Work out the finished part from the listing and answer in its coordinate system (mm). A direction names the side the tool comes from. Coordinates: 2 decimals unless noted, no trailing zeros. Loops run counter-clockwise (first coordinate to the right, second up) from the corner with the lowest first, then second, coordinate; pieces in that order, holes last. Notation, with made-up numbers: (13.25, 26) -> (46.25, 26) arc R6 cw to (46.25, 33) -> close; hole circle Ø9 at (-36, 35.5). An arc over 180 degrees is marked (long way). Use a Markdown table: item, result.
from build123d import *

# Parameters (mm, degrees)
SKETCH_1_R                   = 8
EXTRUDE_1_DEPTH              = 32
SKETCH_2_W                   = 1
SKETCH_2_H                   = 10
CUT_EXTRUDE_2_DEPTH          = 9.25
HOLE_WIZARD_M8_1_D           = 6.8
HOLE_WIZARD_M8_1_DEPTH       = 19.75
HOLE_WIZARD_M8_1_CBORE_D     = 8
HOLE_WIZARD_M8_1_CBORE_DEPTH = 16
HOLE_WIZARD_M8_1_TIP         = 2.042926105
SKETCH_4_R                   = 5
EXTRUDE_3_DEPTH              = 12
CHAMFER_1_SIZE               = 0.5
SKETCH_5_W                   = 1.5
SKETCH_5_H                   = 0.069985642


with BuildPart() as part:
    # 草图1 → 拉伸1 (new body)
    with BuildSketch(Plane.XY):
        Circle(SKETCH_1_R)
    extrude(amount=EXTRUDE_1_DEPTH)

    # 草图2 → 拉伸2 (cut, symmetric)
    with BuildSketch(Plane(origin=(0, 0, 0), x_dir=(1, 0, 0), z_dir=(0, 1, 0))):
        with Locations((-7.5, -16)):
            Rectangle(SKETCH_2_W, SKETCH_2_H)
        with Locations((7.5, -16)):
            Rectangle(SKETCH_2_W, SKETCH_2_H)
    extrude(amount=CUT_EXTRUDE_2_DEPTH, both=True, mode=Mode.SUBTRACT)

    # M8 螺纹孔1
    with Locations(Plane(origin=(0, 0, 0), x_dir=(-1, 0, 0), z_dir=(0, 0, -1))):
        with Locations((0, 0)):
            CounterBoreHole(HOLE_WIZARD_M8_1_D / 2, HOLE_WIZARD_M8_1_CBORE_D / 2, HOLE_WIZARD_M8_1_CBORE_DEPTH, depth=HOLE_WIZARD_M8_1_DEPTH)
            with Locations((0, 0, -(HOLE_WIZARD_M8_1_DEPTH + HOLE_WIZARD_M8_1_TIP / 2))):  # 118° drill point
                Cone(0, HOLE_WIZARD_M8_1_D / 2, HOLE_WIZARD_M8_1_TIP, mode=Mode.SUBTRACT)

    # 草图4 → 拉伸3 (add)
    with BuildSketch(Plane.XY.offset(32)):
        Circle(SKETCH_4_R)
    extrude(amount=EXTRUDE_3_DEPTH)

    # 倒角1
    chamfer_1_edges = [part.edges().sort_by_distance(p)[0] for p in [
        (-5, 0, 44),
    ]]
    chamfer(chamfer_1_edges, length=CHAMFER_1_SIZE)

    # 草图5 → 切除-旋转1 (revolve, cut)
    with BuildSketch(Plane(origin=(0, 0, 0), x_dir=(0, 0, -1), z_dir=(1, 0, 0)), mode=Mode.PRIVATE) as cut_revolve_1_sk:
        with Locations((-32.75, 4.465007179)):
            Rectangle(SKETCH_5_W, SKETCH_5_H)
    revolve(cut_revolve_1_sk.sketch.rotate(Axis((0, 0, 32), (0, 0, -1)), 90), axis=Axis((0, 0, 32), (0, 0, -1)), mode=Mode.SUBTRACT)


solid = part.part
Q1. Section B-B on y = 1.5 is taken. State how many separate pieces and enclosed holes the cut face has, and give its area (3 significant figures).
Solved:
| item | result |
|---|---|
| separate pieces | 1 |
| enclosed holes | 2 |
| area | 454 mm² |
Q2. For faces 5 (the cylindrical face through (0.867, -3.905, 7.888)), 6 (the cylindrical face through (-1.08, -4.88, 37.67)), 7 (the flat face through (-4, -2, 0)), 8 (the flat face through (7.4, 0.1, 21)), 9 (the flat face through (-7.4, -0.1, 21)), determine the directions among +Z, -Z, +X, -X, +Y, -Y from which every point of the face is accessible in a straight line to the end or side of a thin tool.
Solved:
| item | result |
|---|---|
| face 5 | -Z |
| face 6 | +Z |
| face 7 | -Z, +X, -X, +Y, -Y |
| face 8 | +X, +Y, -Y |
| face 9 | -X, +Y, -Y |
Q3. Consider line 1 (Y direction, x = 0, z = 17.2); line 2 (Y direction, x = 0, z = 4); line 3 (Z direction, x = 6, y = 1.25). Determine where each line is inside the solid, lowest interval first. Write a range as [from, to].
Solved:
| item | result |
|---|---|
| line 1 | [-8, -3.4], [3.4, 8] |
| line 2 | [-8, -4], [4, 8] |
| line 3 | [0, 32] |
Q4. Section C-C on z = 38 is taken. Determine the outline of the cut face in (x, y).
Solved:
| item | result |
|---|---|
| outline | circle Ø10 at (0, 0) |
Q5. Determine the mould class of faces 1 (the flat face through (-7.4, -0.1, 11)), 2 (the cylindrical face through (-6.349, -4.868, 15.776)), 3 (the flat face through (7, 0, 16)), 4 (the cylindrical face through (-0.74, -3.32, 17.9)) for opening direction X: pulls with the +X half, pulls with the -X half, needs draft (parallel to the pull), parting line crosses it, or undercut.
Solved:
| item | result |
|---|---|
| face 1 | needs draft |
| face 2 | parting line crosses it |
| face 3 | pulls with the +X half |
| face 4 | undercut |
Q6. Section A-A on z = 12.5 is taken. Determine the outline of the cut face in (x, y).
Solved:
| item | result |
|---|---|
| outline | (-7, -3.87) arc R8 ccw to (7, -3.87) -> (7, 3.87) arc R8 ccw to (-7, 3.87) -> close; hole circle Ø8 at (0, 0) |
Q7. Given pin 1 Ø2 at (x, z) = (5.5, 9) entering from +Y; pin 2 Ø6.5 at (x, y) = (0, 0) entering from -Z; pin 3 Ø4.5 at (x, y) = (0, -1.5) entering from -Z, each flat-ended and moving along its own axis, determine where each tip first touches the part or whether it passes through.
Solved:
| item | result |
|---|---|
| pin 1 | y = 6.61 |
| pin 2 | z = 19.84 |
| pin 3 | z = 16 |
